Read the model definition and answer for the solid it produces. Units are mm, in the model's axes. A direction names the side the tool comes from. Coordinates: 2 decimals unless noted, no trailing zeros. Loops run counter-clockwise (first coordinate to the right, second up) from the corner with the lowest first, then second, coordinate; pieces in that order, holes last. Notation, with made-up numbers: (17.25, 61) -> (48.25, 61) arc R8 cw to (48.25, 65) -> close; hole circle Ø8 at (12.25, -22). An arc over 180 degrees is marked (long way). Answer as a JSON object with one key per item and string values. Group by question number.
Q1. Determine the mould class of faces 1 (the flat face through (2, 13.5, 0)), 2 (the cylindrical face through (1.73, 52.79, 17.72)), 3 (the cylindrical face through (17.93, 29.69, 4.73)) for opening direction Z: released by +Z, released by -Z, zero draft, split by the parting line, or undercut.
Q2. The part is cut by section A-A on y = 39.5. Write down the section's boundary in (x, z) (3 decimals).
Q3. The part is cut by section B-B on x = 17.25. Write down the section's boundary in (y, z) (3 decimals).
Q4. Each of these flat-tipped pins is pushed along its axis until it touches: P1, Ø3, axis at x = 2, z = 0.5, coming from the -Y side; P2, Ø1.6, axis at x = 5, z = -9, coming from the +Y side; P3, Ø2.5, axis at x = 17.25, y = 31, coming from the +Z side; P4, Ø6, axis at x = 7, z = -9, coming from the -Y side. Where does it stop, or does it pass through?
Q5. Straight lines are drawn through the part: line 1 along Z through (x, y) = (15.5, 37) (3 decimals); line 2 along Z through (x, y) = (19, 32) (3 decimals); line 3 along Y through (x, z) = (9.25, -7) (3 decimals). For each, find the intervals that lie inside material, in ascending order. Write a range as [from, to].
Q6. For faces 4 (the flat face through (19.376, 29.618, -11.514)), 5 (the cylindrical face through (1.73, 53.21, 6.28)), 6 (the flat face through (6.643, 39.392, -11.196)), determine the directions among +Z, -Z, +X, -X, +Y, -Y from which every point of the face is accessible in a straight line to the end or side of a thin tool.
Q7. The part is cut by section C-C on x = 6.5. State how many separate pieces and enclosed holes the cut face has, and give its area (3 significant figures).
Q8. The part is cut by section D-D on y = 29. Write down the section's boundary in (x, z) (3 decimals).
from build123d import *

# Parameters (mm, degrees)
F0_R          = 2.5
F1_DEPTH      = 3.5
F0_W          = 5.5
F0_H          = 4
F2_DEPTH      = 25
F4_DEPTH      = 47.001
F5_R          = 1.475
F6_DEPTH      = 16.001
F6_DEPTH_BACK = 19.526
F8_R          = 1.475
F9_DEPTH      = 6.476


with BuildPart() as f1:
    # F0 (on Right) → F1 (new body)
    with BuildSketch(Plane.YZ):
        with BuildLine():
            Line((48.5, -15), (48.5, -16))
            ThreePointArc((48.5, -16), (52.7426406871, -14.2426406871), (54.5, -10))
            ThreePointArc((54.5, -10), (53.2434164903, -6.3257653858), (50, -4.1905249807))
            ThreePointArc((50, -4.1905249807), (48.9188611699, -3.478778179), (48.5, -2.2540333076))
            Line((48.5, -2.2540333076), (48.5, 2.2540333076))
            ThreePointArc((48.5, 2.2540333076), (48.9188611699, 3.478778179), (50, 4.1905249807))
            ThreePointArc((50, 4.1905249807), (53.2434164903, 6.3257653858), (54.5, 10))
            Line((54.5, 10), (54.5, 13.525))
            ThreePointArc((54.5, 13.525), (52.7426406871, 17.7676406871), (48.5, 19.525))
            Line((48.5, 19.525), (48.5, 16.025))
            Line((48.5, 16.025), (13.5, 16.025))
            Line((13.5, 16.025), (13.5, 19.525))
            ThreePointArc((13.5, 19.525), (9.2573593129, 17.7676406871), (7.5, 13.525))
            Line((7.5, 13.525), (7.5, 10))
            ThreePointArc((7.5, 10), (8.7565835097, 6.3257653858), (12, 4.1905249807))
            ThreePointArc((12, 4.1905249807), (13.0811388301, 3.478778179), (13.5, 2.2540333076))
            Line((13.5, 2.2540333076), (13.5, -2.2540333076))
            ThreePointArc((13.5, -2.2540333076), (13.0811388301, -3.478778179), (12, -4.1905249807))
            ThreePointArc((12, -4.1905249807), (8.7565835097, -6.3257653858), (7.5, -10))
            ThreePointArc((7.5, -10), (9.2573593129, -14.2426406871), (13.5, -16))
            Line((13.5, -16), (13.5, -15))
            ThreePointArc((13.5, -15), (8.8970118401, -8.047437581), (17.0950486784, -6.525))
            Line((17.0950486784, -6.525), (44.9049513216, -6.525))
            ThreePointArc((44.9049513216, -6.525), (50.3741340144, -5.3645257313), (53.5, -10))
            ThreePointArc((53.5, -10), (52.0355339059, -13.5355339059), (48.5, -15))
        make_face()
        with BuildLine():
            ThreePointArc((44.9539634802, 6.475), (46.5934563471, 14.6222387757), (53.5, 10))
            ThreePointArc((53.5, 10), (52.0355339059, 6.4644660941), (48.5, 5))
            Line((48.5, 5), (48.5, 3.025))
            Line((48.5, 3.025), (13.5, 3.025))
            Line((13.5, 3.025), (13.5, 5))
            ThreePointArc((13.5, 5), (9.9644660941, 13.5355339059), (18.5, 10))
            ThreePointArc((18.5, 10), (18.1222387757, 8.0934563471), (17.0460365198, 6.475))
            Line((17.0460365198, 6.475), (27.575, 6.475))
            Line((27.575, 6.475), (34.425, 6.475))
            Line((34.425, 6.475), (44.9539634802, 6.475))
        make_face(mode=Mode.SUBTRACT)
        with BuildLine():
            ThreePointArc((48.5, 5), (52.0355339059, 6.4644660941), (53.5, 10))
            ThreePointArc((53.5, 10), (46.5934563471, 14.6222387757), (44.9539634802, 6.475))
            Line((44.9539634802, 6.475), (48.5, 6.475))
            Line((48.5, 6.475), (48.5, 5))
        make_face()
        with Locations((48.5, 10)):
            Circle(F0_R, mode=Mode.SUBTRACT)
        with BuildLine():
            Line((13.5, 6.475), (17.0460365198, 6.475))
            ThreePointArc((17.0460365198, 6.475), (18.1222387757, 8.0934563471), (18.5, 10))
            ThreePointArc((18.5, 10), (9.9644660941, 13.5355339059), (13.5, 5))
            Line((13.5, 5), (13.5, 6.475))
        make_face()
        with Locations((13.5, 10)):
            Circle(F0_R, mode=Mode.SUBTRACT)
        with BuildLine():
            Line((48.5, -14.025), (48.5, -15))
            ThreePointArc((48.5, -15), (52.0355339059, -13.5355339059), (53.5, -10))
            ThreePointArc((53.5, -10), (50.3741340144, -5.3645257313), (44.9049513216, -6.525))
            Line((44.9049513216, -6.525), (48.5, -6.525))
            Line((48.5, -6.525), (48.5, -7.5))
            ThreePointArc((48.5, -7.5), (50.267766953, -8.232233047), (51, -10))
            ThreePointArc((51, -10), (50.267766953, -11.767766953), (48.5, -12.5))
            Line((48.5, -12.5), (48.5, -14.025))
        make_face()
        with BuildLine():
            ThreePointArc((17.0950486784, -6.525), (8.8970118401, -8.047437581), (13.5, -15))
            Line((13.5, -15), (13.5, -14.025))
            Line((13.5, -14.025), (13.5, -12.5))
            ThreePointArc((13.5, -12.5), (11, -10), (13.5, -7.5))
            Line((13.5, -7.5), (13.5, -6.525))
            Line((13.5, -6.525), (17.0950486784, -6.525))
        make_face()
        with BuildLine():
            ThreePointArc((44.9049513216, -6.525), (43.5174738282, -10.4176517058), (45.5336259508, -14.025))
            Line((45.5336259508, -14.025), (48.5, -14.025))
            Line((48.5, -14.025), (48.5, -12.5))
            ThreePointArc((48.5, -12.5), (46, -10), (48.5, -7.5))
            Line((48.5, -7.5), (48.5, -6.525))
            Line((48.5, -6.525), (44.9049513216, -6.525))
        make_face()
        with BuildLine():
            ThreePointArc((18.5, -10), (18.1354742687, -8.1258659856), (17.0950486784, -6.525))
            Line((17.0950486784, -6.525), (13.5, -6.525))
            Line((13.5, -6.525), (13.5, -7.5))
            ThreePointArc((13.5, -7.5), (15.267766953, -8.232233047), (16, -10))
            ThreePointArc((16, -10), (15.267766953, -11.767766953), (13.5, -12.5))
            Line((13.5, -12.5), (13.5, -14.025))
            Line((13.5, -14.025), (16.4663740492, -14.025))
            ThreePointArc((16.4663740492, -14.025), (17.9627273189, -12.2547871023), (18.5, -10))
        make_face()
        with BuildLine():
            ThreePointArc((13.5, 5), (15.420286437, 5.3834536718), (17.0460365198, 6.475))
            Line((17.0460365198, 6.475), (13.5, 6.475))
            Line((13.5, 6.475), (13.5, 5))
        make_face()
        with BuildLine():
            Line((48.5, 6.475), (44.9539634802, 6.475))
            ThreePointArc((44.9539634802, 6.475), (46.579713563, 5.3834536718), (48.5, 5))
            Line((48.5, 5), (48.5, 6.475))
        make_face()
        with BuildLine():
            ThreePointArc((45.5336259508, -14.025), (46.9387505004, -14.75), (48.5, -15))
            Line((48.5, -15), (48.5, -14.025))
            Line((48.5, -14.025), (45.5336259508, -14.025))
        make_face()
        with BuildLine():
            Line((13.5, -14.025), (13.5, -15))
            ThreePointArc((13.5, -15), (15.0612494996, -14.75), (16.4663740492, -14.025))
            Line((16.4663740492, -14.025), (13.5, -14.025))
        make_face()
    extrude(amount=F1_DEPTH)

    # F0 (on Right) → F2 (join)
    with BuildSketch(Plane.YZ):
        with Locations((31, -12.025)):
            Rectangle(F0_W, F0_H)
        with BuildLine():
            ThreePointArc((48.5, 5), (46.579713563, 5.3834536718), (44.9539634802, 6.475))
            Line((44.9539634802, 6.475), (34.425, 6.475))
            Line((34.425, 6.475), (27.575, 6.475))
            Line((27.575, 6.475), (17.0460365198, 6.475))
            ThreePointArc((17.0460365198, 6.475), (15.420286437, 5.3834536718), (13.5, 5))
            Line((13.5, 5), (13.5, 3.025))
            Line((13.5, 3.025), (48.5, 3.025))
            Line((48.5, 3.025), (48.5, 5))
        make_face()
        Polygon((48.5, 16.025), (48.5, 19.525), (35.4, 19.525), (26.6, 19.525), (13.5, 19.525), (13.5, 16.025), align=None)
        with BuildLine():
            Line((33.75, -14.025), (45.5336259508, -14.025))
            ThreePointArc((45.5336259508, -14.025), (43.5174738282, -10.4176517058), (44.9049513216, -6.525))
            Line((44.9049513216, -6.525), (17.0950486784, -6.525))
            ThreePointArc((17.0950486784, -6.525), (18.1354742687, -8.1258659856), (18.5, -10))
            ThreePointArc((18.5, -10), (17.9627273189, -12.2547871023), (16.4663740492, -14.025))
            Line((16.4663740492, -14.025), (28.25, -14.025))
            Line((28.25, -14.025), (28.25, -10.025))
            Line((28.25, -10.025), (33.75, -10.025))
            Line((33.75, -10.025), (33.75, -14.025))
        make_face()
        with BuildLine():
            Line((13.5, -16), (48.5, -16))
            Line((48.5, -16), (48.5, -15))
            ThreePointArc((48.5, -15), (46.9387505004, -14.75), (45.5336259508, -14.025))
            Line((45.5336259508, -14.025), (33.75, -14.025))
            Line((33.75, -14.025), (28.25, -14.025))
            Line((28.25, -14.025), (16.4663740492, -14.025))
            ThreePointArc((16.4663740492, -14.025), (15.0612494996, -14.75), (13.5, -15))
            Line((13.5, -15), (13.5, -16))
        make_face()
    extrude(amount=F2_DEPTH)

    # F3 (on face) → F4 (cut, through all)
    with BuildSketch(Plane(origin=(0, 54.5, 0), x_dir=(-1, 0, 0), z_dir=(0, 1, 0))):
        Polygon((-25, -12.525), (-25, -16), (-3.5, -16), align=None)
    extrude(amount=-F4_DEPTH, mode=Mode.SUBTRACT)

    # F5 (on Top) → F6 (cut, two sides)
    with BuildSketch(Plane.XY) as f6_sk:
        with BuildLine():
            ThreePointArc((20.7938548449, 35.8416002353), (23.25, 31), (20.7938548449, 26.1583997647))
            Line((20.7938548449, 26.1583997647), (3.5, 13.5))
            Line((3.5, 13.5), (25, 13.5))
            Line((25, 13.5), (25, 48.5))
            Line((25, 48.5), (3.5, 48.5))
            Line((3.5, 48.5), (20.7938548449, 35.8416002353))
        make_face()
        with Locations((17.25, 31)):
            Circle(F5_R)
        with BuildLine():
            Line((9.6998989998, 37.7656271516), (3.5, 41.0644418683))
            Line((3.5, 41.0644418683), (3.5, 34))
            Line((3.5, 34), (8.7604519489, 34))
            ThreePointArc((8.7604519489, 34), (10.7009743403, 35.5158793039), (9.6998989998, 37.7656271516))
        make_face()
        with BuildLine():
            Line((3.5, 28), (3.5, 20.9355581317))
            Line((3.5, 20.9355581317), (9.6998989998, 24.2343728484))
            ThreePointArc((9.6998989998, 24.2343728484), (10.7009743403, 26.4841206961), (8.7604519489, 28))
            Line((8.7604519489, 28), (3.5, 28))
        make_face()
    extrude(amount=-F6_DEPTH, mode=Mode.SUBTRACT)
    extrude(f6_sk.sketch, amount=F6_DEPTH_BACK, mode=Mode.SUBTRACT)

    # F8 (on offset) → F9 (cut, through all)
    with BuildSketch(Plane.XY.offset(-9.525)):
        Polygon((20.173566383, 31), (18.6002868994, 33.725), (15.4537279323, 33.725), (13.8804484488, 31), (15.4537279323, 28.275), (18.6002868994, 28.275), align=None)
        with Locations((17.25, 31)):
            Circle(F8_R, mode=Mode.SUBTRACT)
    extrude(amount=-F9_DEPTH, mode=Mode.SUBTRACT)


solid = f1.part
Final values:
{
 "1": {"face 1": "undercut", "face 2": "released by +Z", "face 3": "zero draft"},
 "2": {"outline": "(0, -16) -> (3.5, -16) -> (3.5, 19.525) -> (0, 19.525) -> close; (6.44, -15.525) -> (15.796, -14.013) -> (15.796, -6.525) -> (6.44, -6.525) -> close; (6.44, 3.025) -> (15.796, 3.025) -> (15.796, 6.475) -> (6.44, 6.475) -> close; (6.44, 16.025) -> (15.796, 16.025) -> (15.796, 19.525) -> (6.44, 19.525) -> close"},
 "3": {"outline": "(23.564, -13.778) -> (28.275, -13.778) -> (28.275, -9.525) -> (29.525, -9.525) -> (29.525, -6.525) -> (23.564, -6.525) -> close; (23.564, 3.025) -> (29.525, 3.025) -> (29.525, 6.475) -> (23.564, 6.475) -> close; (23.564, 16.025) -> (29.525, 16.025) -> (29.525, 19.525) -> (23.564, 19.525) -> close; (32.475, -9.525) -> (33.725, -9.525) -> (33.725, -13.778) -> (38.436, -13.778) -> (38.436, -6.525) -> (32.475, -6.525) -> close; (32.475, 3.025) -> (38.436, 3.025) -> (38.436, 6.475) -> (32.475, 6.475) -> close; (32.475, 16.025) -> (38.436, 16.025) -> (38.436, 19.525) -> (32.475, 19.525) -> close"},
 "4": {"P1": "stops at y = 13.5", "P2": "stops at y = 43.84", "P3": "passes through", "P4": "stops at y = 17.1"},
 "5": {"line 1": "z = [-14.06, -6.525], [3.025, 6.475], [16.025, 19.525]", "line 2": "z = [-9.525, -6.525], [3.025, 6.475], [16.025, 19.525]", "line 3": "y = [17.709, 23.995], [27.939, 34.061], [38.005, 44.291]"},
 "6": {"face 4": "-Z", "face 5": "+X, -X, +Y", "face 6": "+Z, -Z"},
 "7": {"separate pieces": "9", "enclosed holes": "0", "area": "278 mm2"},
 "8": {"outline": "(0, -16) -> (3.5, -16) -> (15.035, -14.136) -> (15.035, -9.525) -> (19.019, -9.525) -> (19.019, -13.492) -> (22.907, -12.863) -> (22.907, -6.525) -> (3.5, -6.525) -> (3.5, 3.025) -> (22.907, 3.025) -> (22.907, 6.475) -> (3.5, 6.475) -> (3.5, 16.025) -> (22.907, 16.025) -> (22.907, 19.525) -> (0, 19.525) -> close"}
}
